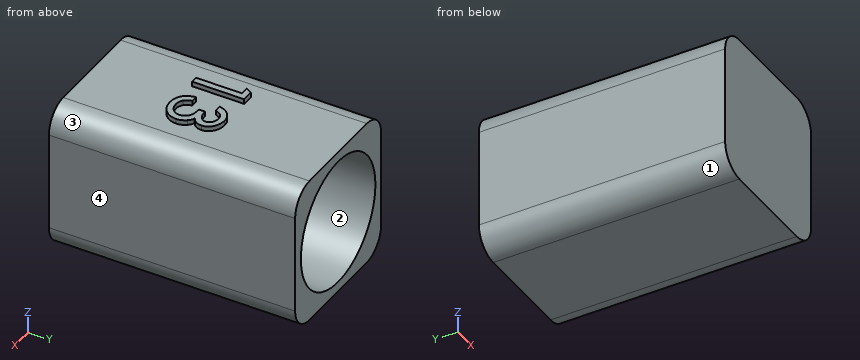
```python
from build123d import *

# Parameters (mm, degrees)
SKETCH1_W           = 15
SKETCH1_H           = 15
BOSS_EXTRUDE1_DEPTH = 25
SKETCH2_R           = 6.5
CUT_EXTRUDE1_DEPTH  = 24
BOSS_EXTRUDE3_DEPTH = 0.5
FILLET1_R           = 2.5
FILLET2_R           = 2.5
FILLET3_R           = 2.5
FILLET4_R           = 2.5


with BuildPart() as part:
    # Sketch1 → Boss-Extrude1 (new body)
    with BuildSketch(Plane(origin=(0, 0, 0), x_dir=(1, 0, 0), z_dir=(0, 1, 0))):
        Rectangle(SKETCH1_W, SKETCH1_H)
    extrude(amount=BOSS_EXTRUDE1_DEPTH)

    # Sketch2 → Cut-Extrude1 (cut)
    with BuildSketch(Plane(origin=(0, 25, 0), x_dir=(1, 0, 0), z_dir=(0, 1, 0))):
        with Locations(Location((0, 0, 0), (0, 0, 270))):
            Circle(SKETCH2_R)
    extrude(amount=-CUT_EXTRUDE1_DEPTH, mode=Mode.SUBTRACT)

    # Sketch3 → Boss-Extrude3 (add)
    with BuildSketch(Plane.XY.offset(7.5)):
        Polygon((-3.300679086, 14.210073329), (-2.149487179, 14.210073329), (-2.149487179, 8.918406662), (-2.827905982, 8.918406662), (-2.827905982, 13.599496406), (-3.642008546, 13.599496406), align=None)
        with BuildLine():
            Line((0.536627271, 12.921077603), (-0.114230768, 12.921077603))
            add(Edge.make_bspline(
                [(-0.114230768, 12.921077603), (-0.100961493, 12.97960801), (-0.074987112, 13.094180286), (-0.022481053, 13.257850992), (0.036681085, 13.410915565), (0.105032166, 13.552204246), (0.18423708, 13.680615371), (0.269979947, 13.798627118), (0.365943067, 13.903778446), (0.470019389, 13.997523947), (0.581683486, 14.078506256), (0.697631037, 14.150346176), (0.818785512, 14.210579109), (0.944384477, 14.26104525), (1.07507306, 14.299243023), (1.210742775, 14.325043417), (1.350596953, 14.343167819), (1.445719829, 14.344887341), (1.493833802, 14.34575709)],
                knots=[0, 0, 0, 0, 1.225194122, 2.398296627, 3.506547767, 4.574817873, 5.598350885, 6.584148364, 7.54966307, 8.500147383, 9.439776218, 10.36307994, 11.282851771, 12.199447467, 13.124300948, 14.058371117, 15.017907346, 16, 16, 16, 16], degree=3))
            add(Edge.make_bspline(
                [(1.493833802, 14.34575709), (1.568531598, 14.343241617), (1.716386062, 14.338262569), (1.934195583, 14.30064004), (2.143451442, 14.236059647), (2.342206832, 14.148760529), (2.525877316, 14.041870431), (2.688320429, 13.917169074), (2.828024385, 13.777755988), (2.940950824, 13.623466287), (3.030374612, 13.461564399), (3.094266969, 13.295358681), (3.134897281, 13.126546953), (3.139755234, 13.012814321), (3.142179488, 12.956058572)],
                knots=[0, 0, 0, 0, 1.126551995, 2.229861531, 3.322496069, 4.422827045, 5.497949776, 6.520418829, 7.504194933, 8.464779191, 9.395175895, 10.286118409, 11.144725379, 12, 12, 12, 12], degree=3))
            add(Edge.make_bspline(
                [(3.142179488, 12.956058572), (3.140445745, 12.901156816), (3.137054029, 12.793752712), (3.107562398, 12.637619364), (3.060141337, 12.491151022), (2.992304739, 12.354955699), (2.905853989, 12.228760675), (2.799194916, 12.113655832), (2.674433691, 12.007543566), (2.580108351, 11.947900553), (2.531602565, 11.917229779)],
                knots=[0, 0, 0, 0, 1.039530957, 2.033630564, 2.999111873, 3.948297759, 4.906578666, 5.887513816, 6.913676835, 8, 8, 8, 8], degree=3))
            add(Edge.make_bspline(
                [(2.531602565, 11.917229779), (2.584015029, 11.894773533), (2.688596929, 11.849965164), (2.830947045, 11.754438191), (2.961806101, 11.640433311), (3.034980771, 11.549892367), (3.072217549, 11.503818321)],
                knots=[0, 0, 0, 0, 0.990740455, 1.976887035, 2.970487876, 4, 4, 4, 4], degree=3))
            add(Edge.make_bspline(
                [(3.072217549, 11.503818321), (3.099199896, 11.466345), (3.152494918, 11.392328407), (3.223193721, 11.27672227), (3.280661614, 11.15750979), (3.330599467, 11.03769875), (3.36747824, 10.915047449), (3.394052073, 10.790627171), (3.410528936, 10.664010495), (3.412537758, 10.578814684), (3.413547009, 10.536011497)],
                knots=[0, 0, 0, 0, 1.060434252, 2.094549648, 3.107169572, 4.097295716, 5.072846837, 6.043796276, 7.017184609, 8, 8, 8, 8], degree=3))
            add(Edge.make_bspline(
                [(3.413547009, 10.536011497), (3.410884478, 10.462255283), (3.405544113, 10.314318949), (3.355756698, 10.095274277), (3.279517444, 9.87949602), (3.190263242, 9.706554209), (3.106229875, 9.572451392), (3.035363238, 9.476738788), (2.959072469, 9.385890858), (2.875352239, 9.302061826), (2.786861322, 9.222237669), (2.690771017, 9.149101484), (2.588777456, 9.08119272), (2.481373466, 9.018753249), (2.368425447, 8.963923848), (2.25238329, 8.914613155), (2.131846342, 8.875070384), (2.009065285, 8.840230397), (1.881992689, 8.815601905), (1.751948266, 8.795813187), (1.618014874, 8.78571627), (1.527767864, 8.783727609), (1.482173479, 8.782722902)],
                knots=[0, 0, 0, 0, 1.521749033, 3.052244174, 4.617626532, 6.240122497, 7.060311358, 7.885196768, 8.698339091, 9.508724546, 10.330730427, 11.158549718, 12.000758621, 12.860902525, 13.722748307, 14.593084173, 15.463328201, 16.341708233, 17.227848997, 18.135261118, 19.057900949, 20, 20, 20, 20], degree=3))
            add(Edge.make_bspline(
                [(1.482173479, 8.782722902), (1.424534496, 8.784009629), (1.311091495, 8.786542119), (1.144761754, 8.80453533), (0.985505782, 8.835279516), (0.833832902, 8.878940615), (0.688754462, 8.933826723), (0.551698785, 9.002209379), (0.421541769, 9.081928184), (0.298933599, 9.17442013), (0.185538343, 9.280567865), (0.081506968, 9.400204964), (-0.010374271, 9.534920483), (-0.093429441, 9.682647813), (-0.165387817, 9.845073744), (-0.2274602, 10.020890903), (-0.280102876, 10.210673196), (-0.304959207, 10.342867972), (-0.317756409, 10.41092803)],
                knots=[0, 0, 0, 0, 1.031951552, 2.031050468, 2.99141865, 3.932589319, 4.853771667, 5.764839348, 6.670884665, 7.583203617, 8.509779947, 9.447179227, 10.415909331, 11.424319639, 12.477825485, 13.592421652, 14.760465984, 16, 16, 16, 16], degree=3))
            Line((-0.317756409, 10.41092803), (0.340521836, 10.41092803))
            add(Edge.make_bspline(
                [(0.340521836, 10.41092803), (0.353642264, 10.365961117), (0.378781523, 10.27980274), (0.419994104, 10.156753231), (0.464328654, 10.046178878), (0.510010421, 9.946594394), (0.557269249, 9.858400707), (0.607129332, 9.781740097), (0.658566183, 9.715895757), (0.697291944, 9.679781396), (0.715772237, 9.662547287)],
                knots=[0, 0, 0, 0, 1.326285875, 2.54121601, 3.672658499, 4.697761427, 5.642367002, 6.502616728, 7.285434817, 8, 8, 8, 8], degree=3))
            add(Edge.make_bspline(
                [(0.715772237, 9.662547287), (0.742522938, 9.640711231), (0.795504144, 9.597463744), (0.882749756, 9.543986167), (0.972720363, 9.496111587), (1.068630016, 9.460087268), (1.167568548, 9.429638048), (1.271216907, 9.408640374), (1.37901821, 9.395682345), (1.452455657, 9.394100021), (1.489593684, 9.393299825)],
                knots=[0, 0, 0, 0, 0.989076215, 1.958918776, 2.928708407, 3.907140108, 4.891221483, 5.894723991, 6.935341563, 8, 8, 8, 8], degree=3))
            add(Edge.make_bspline(
                [(1.489593684, 9.393299825), (1.535564055, 9.394385116), (1.625629073, 9.396511414), (1.756948364, 9.411119566), (1.881465881, 9.436816065), (1.998634057, 9.472540053), (2.109229372, 9.518420277), (2.212093691, 9.574823167), (2.308446041, 9.640715678), (2.395915, 9.717176651), (2.474283993, 9.800159305), (2.544168737, 9.886739881), (2.603887301, 9.976492114), (2.651728418, 10.070571325), (2.689422936, 10.167818589), (2.715520817, 10.268504187), (2.732250533, 10.372562903), (2.734159496, 10.443017471), (2.735128206, 10.47876991)],
                knots=[0, 0, 0, 0, 1.196856166, 2.344877135, 3.434653565, 4.502660904, 5.529498559, 6.546397239, 7.551828815, 8.562675341, 9.564818567, 10.520268272, 11.456705045, 12.365995596, 13.262962725, 14.166698094, 15.069683942, 16, 16, 16, 16], degree=3))
            add(Edge.make_bspline(
                [(2.735128206, 10.47876991), (2.733019747, 10.525931359), (2.728805675, 10.620190586), (2.696820658, 10.758793296), (2.645521251, 10.893210689), (2.573056785, 11.020296841), (2.484855208, 11.139353782), (2.379063635, 11.243639788), (2.258444845, 11.332741278), (2.145936485, 11.394343128), (2.04399224, 11.435052667), (1.955096408, 11.463378228), (1.854145901, 11.488537229), (1.741612839, 11.510578276), (1.61711797, 11.529541882), (1.480621111, 11.545196857), (1.331763956, 11.55768696), (1.228486925, 11.5640896), (1.174764958, 11.567420084)],
                knots=[0, 0, 0, 0, 1.058801672, 2.116173898, 3.179133807, 4.280986043, 5.392377071, 6.498225676, 7.604871823, 8.752253925, 9.368447799, 10.068883315, 10.846735517, 11.704571958, 12.644304815, 13.675272135, 14.790738352, 16, 16, 16, 16], degree=3))
            Line((1.174764958, 11.567420084), (1.174764958, 12.174816919))
            add(Edge.make_bspline(
                [(1.174764958, 12.174816919), (1.244792803, 12.176105368), (1.379225183, 12.178578803), (1.572223534, 12.201059455), (1.747870691, 12.237255938), (1.905314059, 12.288971698), (2.042647935, 12.35297773), (2.161778734, 12.421655594), (2.259068443, 12.499974424), (2.335704951, 12.585390944), (2.392038085, 12.677435042), (2.43474333, 12.771757648), (2.458395507, 12.871531566), (2.461961466, 12.938985103), (2.463760685, 12.973019042)],
                knots=[0, 0, 0, 0, 1.49683591, 2.87347434, 4.147795521, 5.325633569, 6.407353164, 7.383009189, 8.25851615, 9.066624807, 9.823413814, 10.557538392, 11.272200497, 12, 12, 12, 12], degree=3))
            add(Edge.make_bspline(
                [(2.463760685, 12.973019042), (2.462989319, 12.998165871), (2.461468952, 13.047730405), (2.447975215, 13.120981745), (2.427069851, 13.191877769), (2.3971723, 13.260279908), (2.358008252, 13.325569974), (2.311713599, 13.389235409), (2.255758848, 13.449820095), (2.192602073, 13.507555086), (2.123479924, 13.561310327), (2.048694297, 13.608437464), (1.969006195, 13.647585237), (1.884409587, 13.67941094), (1.795493257, 13.704957023), (1.701488974, 13.722876037), (1.602919685, 13.73365892), (1.535556151, 13.734666896), (1.501254007, 13.735180167)],
                knots=[0, 0, 0, 0, 0.88508993, 1.744517034, 2.61478088, 3.484243336, 4.365825862, 5.291885516, 6.252189795, 7.265246754, 8.303377192, 9.332440159, 10.373327524, 11.425096702, 12.51242353, 13.62794981, 14.792129802, 16, 16, 16, 16], degree=3))
            add(Edge.make_bspline(
                [(1.501254007, 13.735180167), (1.451999534, 13.733049362), (1.355744815, 13.728885274), (1.215849293, 13.698979708), (1.08596836, 13.646935622), (0.984693576, 13.587633927), (0.908608791, 13.527502106), (0.852738473, 13.471044634), (0.798434832, 13.40397858), (0.743075275, 13.32807166), (0.689987439, 13.24084643), (0.637503486, 13.143811145), (0.585220048, 13.036405205), (0.553221665, 12.960461885), (0.536627271, 12.921077603)],
                knots=[0, 0, 0, 0, 1.30644707, 2.553102055, 3.773430717, 5.004978473, 5.652102429, 6.34150733, 7.107309491, 7.939915375, 8.832283585, 9.813897121, 10.866284818, 12, 12, 12, 12], degree=3))
        make_face()
    extrude(amount=BOSS_EXTRUDE3_DEPTH)

    # Fillet1
    fillet1_edges = [part.edges().sort_by_distance(p)[0] for p in [
        (-7.5, 12.5, 7.5),
    ]]
    fillet(fillet1_edges, radius=FILLET1_R)

    # Fillet2
    fillet2_edges = [part.edges().sort_by_distance(p)[0] for p in [
        (7.5, 12.5, 7.5),
    ]]
    fillet(fillet2_edges, radius=FILLET2_R)

    # Fillet3
    fillet3_edges = [part.edges().sort_by_distance(p)[0] for p in [
        (7.5, 12.5, -7.5),
    ]]
    fillet(fillet3_edges, radius=FILLET3_R)

    # Fillet4
    fillet4_edges = [part.edges().sort_by_distance(p)[0] for p in [
        (-7.5, 12.5, -7.5),
    ]]
    fillet(fillet4_edges, radius=FILLET4_R)


solid = part.part
```
Work out the finished part from the listing and answer in its coordinate system (mm). Face numbers are marked on the shaded views. Give positions to 0.01 mm unless a question says otherwise; leave off trailing zeros. Order: outer loops, then holes, each group sorted by start corner. A loop starts at its lowest first (then second) coordinate and runs counter-clockwise, first axis right, second up.
1. Section B-B, the plane z = 0 is taken. Determine the outline of the cut face in (x, y), and give its area (3 significant figures).
Result sheet:
outline: (-7.5, 0) - (7.5, 0) - (7.5, 25) - (6.5, 25) - (6.5, 1) - (-6.5, 1) - (-6.5, 25) - (-7.5, 25) - close
area: 63.0 mm2
2. Straight lines are drawn through the part: L1, parallel to X at y = 12.75, z = 0; L2, parallel to Y at x = -4, z = 3.5; L3, parallel to Z at x = -2.25, y = 22.5. For each, find the intervals that lie inside material, in ascending order.
Result sheet:
L1: x = -7.5 to -6.5, 6.5 to 7.5
L2: y = 0 to 1
L3: z = -7.5 to -6.1, 6.1 to 7.5
3. The mould has two halves that part along Z. Classify the marked faces 1, 2, 3 and 4: released by +Z, released by -Z, zero draft, split by the parting line, or undercut.
Result sheet:
face 1: released by -Z
face 2: undercut
face 3: released by +Z
face 4: zero draft
4. Section C-C, the plane x = 5.5 is taken. Determine the outline of the cut face in (y, z), and give its area (3 significant figures).
Result sheet:
outline: (0, -7.45) - (25, -7.45) - (25, -3.46) - (1, -3.46) - (1, 3.46) - (25, 3.46) - (25, 7.45) - (0, 7.45) - close
area: 206 mm2
5. Each of these flat-tipped pins is pushed along its axis until it touches: P1, Ø4, axis at y = 16.5, z = 6.5, coming from the -X side; P2, Ø4, axis at x = -1.5, z = -2, coming from the +Y side. Where does it stop, or does it pass through?
Result sheet:
P1: stops at x = -7.5
P2: stops at y = 1
6. Section A-A, the plane y = 16.75 is taken. Determine the outline of the cut face in (x, z), and give its area (3 significant figures).
Result sheet:
outline: (-7.5, -5) arc R2.5 ccw to (-5, -7.5) - (5, -7.5) arc R2.5 ccw to (7.5, -5) - (7.5, 5) arc R2.5 ccw to (5, 7.5) - (-5, 7.5) arc R2.5 ccw to (-7.5, 5) - close; hole circle Ø13 at (0, 0)
area: 86.9 mm2
